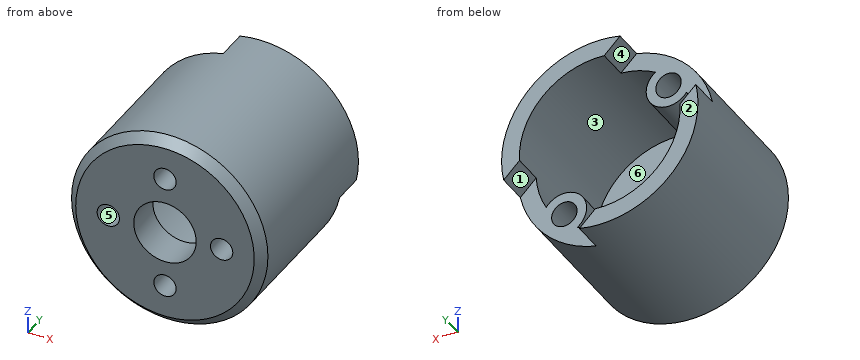
Autodesk Inventor part; units mm, degrees
ref_plane "YZ Plane" through (0, 0, 0) normal (1, 0, 0) x (0, 1, 0)
ref_plane "XZ Plane" through (0, 0, 0) normal (0, 1, 0) x (-1, 0, 0)
ref_plane "XY Plane" through (0, 0, 0) normal (0, 0, 1) x (1, 0, 0)
sketch "Esboço1" plane through (0, 0, 0) normal (0, 0, 1) x (1, 0, 0)
  line L0 (-9, 20) -> (-9, 4)
  line L1 (-9, 4) -> (0, 4)
  line L2 (0, 4) -> (0, 0)
  line L3 (0, 0) -> (-10, 0)
  line L4 (-11, 1) -> (-11, 20)
  line L5 (-11, 1) -> (-10, 0)
  line L6 (-11, 20) -> (-9, 20)
  dimension "d0" = 18
  dimension "d1" = 2
  dimension "d2" = 4
  dimension "d10" = 45
  dimension "d11" = 1
  dimension "d30" = 20
revolve "Revolução1" add sketch "Esboço1" angle 360 about axis through (0, 4, 0) along (0, -1, 0)
sketch "Esboço2" plane through (0, 4, 0) normal (0, 1, 0) x (1, 0, 0)
  circle A0 centre (0, 0) radius 3.5
  circle A1 centre (0, 0) radius 6.35 construction
  circle A2 centre (0, 6.35) radius 1.25
  circle A3 centre (0, -6.35) radius 1.25
  circle A4 centre (-6.35, 0) radius 1.25
  circle A5 centre (6.35, 0) radius 1.25
  circle A6 centre (0, 6.35) radius 2.5
  dimension "d12" = 7
  dimension "d13" = 12.7
  dimension "d14" = 2.5
  dimension "d48" = 5
extrude "Extrusão1" cut sketch "Esboço2" against normal through all contours A0 | A2 | A3 | A4 | A5
sketch "Esboço5" plane through (0, 20, 0) normal (0, 1, 0) x (1, 0, 0)
  circle A0 centre (0, 0) radius 9
  arc A1 (-4.3758, -7.8646) -> (-7.8646, -4.3758) centre (-5.8336, -5.8336) ccw
  line L0 (-15.4, 0) -> (15.4, 0)
  circle A2 centre (0, 0) radius 8.25 construction
  arc A3 (4.3758, 7.8646) -> (7.8646, 4.3758) centre (5.8336, 5.8336) ccw
  line L1 (-5.8336, -5.8336) -> (5.8336, 5.8336) construction
  dimension "d32" = 2.5
  dimension "d49" = 45
  dimension "d50" = 16.5
extrude "Extrusão4" add sketch "Esboço5" against normal up to surface (16 mm away) contours A3 A0 | A0 A1
sketch "Esboço7" plane through (0, 20, 0) normal (0, 1, 0) x (1, 0, 0)
  arc A0 (-4.3758, -7.8646) -> (-7.8646, -4.3758) centre (-5.8336, -5.8336) ccw
  arc A1 (4.3758, 7.8646) -> (7.8646, 4.3758) centre (5.8336, 5.8336) ccw
  point P0 (0, 0)
hole "Furo1" at (-5.8336, 20, 5.8336) at (5.8336, 20, -5.8336) direction (0, -1, 0) diameter 2.85 depth 16
sketch "Esboço6" plane through (0, 20, 0) normal (0, 1, 0) x (1, 0, 0)
  circle A0 centre (0, 0) radius 11
  line L0 (2.2766, 10.7618) -> (-10.7618, -2.2766)
  line L1 (10.7618, 2.2766) -> (-2.2766, -10.7618)
  circle A1 centre (0, 0) radius 11
  line L2 (-5.8336, -5.8336) -> (5.8336, 5.8336) construction
  circle A2 centre (-5.8336, -5.8336) radius 1.425
  circle A3 centre (5.8336, 5.8336) radius 1.425
  point P0 (-2.2766, -10.7618)
  dimension "d45" = 12
extrude "Extrusão5" cut sketch "Esboço6" against normal blind 3.5 contours L1 A0 L0 | A2 | A3
properties part number "_3DPrint"
Part model, mm, in its own coordinate system. Face numbers are marked on the shaded views. A direction names the side the tool comes from. Coordinates: 2 decimals unless noted, no trailing zeros. Order: outer loops, then holes, each group sorted by start corner. A loop starts at its lowest first (then second) coordinate and runs counter-clockwise, first axis right, second up. Notation, with made-up numbers: M 57,60 L 105,60 A14 ccw 105,80 Z; hole C 37,-40 d5. An arc over 180 degrees is marked long. Use a Markdown table: item, result.
(1) Flat gauge pins, fed straight in: pin 1 (5 mm diameter, centred on x = -4.5, y = 7.5, fed in from -Z); pin 2 (0.9 mm diameter, centred on x = -5.5, z = 6, fed in from +Y); pin 3 (3 mm diameter, centred on x = 8, z = -6, fed in from +Y). Where does each tip first touch, or does it go through?
A:
| item | result |
|---|---|
| pin 1 | stops at z = -10.82 |
| pin 2 | stops at y = 4 |
| pin 3 | stops at y = 16.5 |
(2) Pull direction Z, two halves, no side cores. Call the marked faces 1, 2 and 3: released by +Z, released by -Z, zero draft, split by the parting line, or undercut.
A:
| item | result |
|---|---|
| face 1 | released by -Z |
| face 2 | zero draft |
| face 3 | undercut |
(3) Probe L1, parallel to X at y = 2.65, z = 0; L2, parallel to Z at x = 0, y = 14. List the from-to ranges inside material, lowest first.
A:
| item | result |
|---|---|
| L1 | x = -11 to -7.6, -5.1 to -3.5, 3.5 to 5.1, 7.6 to 11 |
| L2 | z = -11 to -9, 9 to 11 |
(4) Cut at A-A on z = 0. Write the cut outline in (x, y), then the cut area to 3 significant figures.
A:
| item | result |
|---|---|
| outline | M -11,1 L -10,0 L -7.6,0 L -7.6,4 L -9,4 L -9,20 L -11,20 Z; M -5.1,0 L -3.5,0 L -3.5,4 L -5.1,4 Z; M 3.5,0 L 5.1,0 L 5.1,4 L 3.5,4 Z; M 7.6,0 L 10,0 L 11,1 L 11,20 L 9,20 L 9,4 L 7.6,4 Z |
| area | 103 mm^2 |
(5) Cut at B-B on y = 8. Write the cut outline in (x, z) (3 decimals).
A:
| item | result |
|---|---|
| outline | C 0,0 d22; hole M -7.865,4.376 A9 ccw 4.376,-7.865 A2.5 cw long 7.865,-4.376 A9 ccw -4.376,7.865 A2.5 cw long Z; hole C -5.834,5.834 d2.85; hole C 5.834,-5.834 d2.85 |
(6) Tool access for the marked faces 4, 5 and 6: list every direction of +Z, -Z, +X, -X, +Y, -Y with a clear straight run to the whole face (end or side of a thin tool).
A:
| item | result |
|---|---|
| face 4 | -X, +Y |
| face 5 | +Y, -Y |
| face 6 | +Y |
